Can you work these out from the model? Positions are in its coordinate system, mm. Round coordinates to 2 decimals unless told otherwise and drop trailing zeros. Order: outer loops, then holes, each group sorted by start corner. A loop starts at its lowest first (then second) coordinate and runs counter-clockwise, first axis right, second up.
Q1. If we section it at A-A (y = 68): Please give me the cut outline in (x, z), plus the area to 3 significant figures.
Q2. If we section it at D-D (x = 195): Please give me the cut outline in (y, z), plus the area to 3 significant figures.
Q3. If we section it at C-C (z = 4.5): Count the separate pieces of the cut face and the enclosed holes in it, plus the area to 3 significant figures.
Q4. If we section it at B-B (y = 10): Please give me the cut outline in (x, z).
Q5. If I drill on line 1 (Y direction, x = 30, z = 8.75); line 2 (X direction, y = 150, z = 2.5); line 3 (Y direction, x = 71.5, z = 11.5), over which ranges is the centre line in solid material (lowest first)?
Q6. Will this pin go through, and if not, where does the flat tip stop? P1, Ø3, axis at x = 30, y = 120, coming from the +Z side.
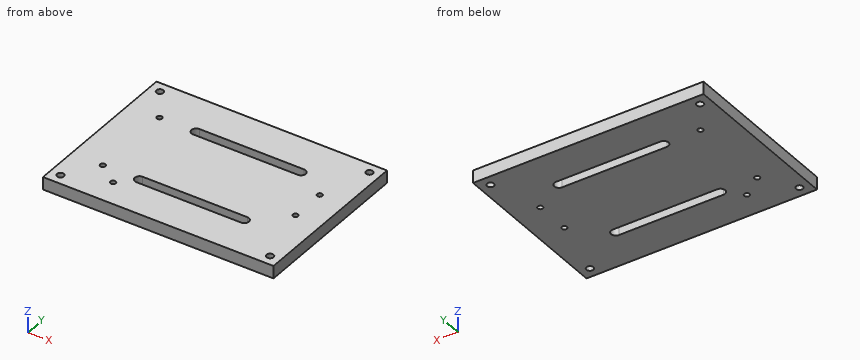
from build123d import *

# Parameters (mm, degrees)
SKETCH_1_W                  = 220
SKETCH_1_H                  = 160
SKETCH_1_R                  = 3.3
SKETCH_1_R_2                = 2.5
BASE_PLATE_220X160X12_DEPTH = 12


with BuildPart() as part:
    # 草图1 → Base_plate_220x160x12 (new body)
    with BuildSketch(Plane.XY):
        with Locations((110, 80)):
            Rectangle(SKETCH_1_W, SKETCH_1_H)
        with Locations((10, 10)):
            Circle(SKETCH_1_R, mode=Mode.SUBTRACT)
        with Locations((10, 150)):
            Circle(SKETCH_1_R, mode=Mode.SUBTRACT)
        with Locations((210, 10)):
            Circle(SKETCH_1_R, mode=Mode.SUBTRACT)
        with Locations((210, 150)):
            Circle(SKETCH_1_R, mode=Mode.SUBTRACT)
        with Locations((30, 40)):
            Circle(SKETCH_1_R_2, mode=Mode.SUBTRACT)
        with Locations((30, 120)):
            Circle(SKETCH_1_R_2, mode=Mode.SUBTRACT)
        with Locations((50, 25)):
            Circle(SKETCH_1_R_2, mode=Mode.SUBTRACT)
        with Locations((195, 68)):
            Circle(SKETCH_1_R_2, mode=Mode.SUBTRACT)
        with Locations((195, 102)):
            Circle(SKETCH_1_R_2, mode=Mode.SUBTRACT)
        with BuildLine():
            Line((65, 44.5), (165, 44.5))
            ThreePointArc((165, 44.5), (169.5, 40), (165, 35.5))
            Line((165, 35.5), (65, 35.5))
            ThreePointArc((65, 35.5), (60.5, 40), (65, 44.5))
        make_face(mode=Mode.SUBTRACT)
        with BuildLine():
            Line((65, 124.5), (165, 124.5))
            ThreePointArc((165, 124.5), (169.5, 120), (165, 115.5))
            Line((165, 115.5), (65, 115.5))
            ThreePointArc((65, 115.5), (60.5, 120), (65, 124.5))
        make_face(mode=Mode.SUBTRACT)
    extrude(amount=BASE_PLATE_220X160X12_DEPTH)


solid = part.part
Solution:
1. outline: (0, 0) - (192.5, 0) - (192.5, 12) - (0, 12) - close; (197.5, 0) - (220, 0) - (220, 12) - (197.5, 12) - close
1. area: 2,580 mm2
2. outline: (0, 0) - (65.5, 0) - (65.5, 12) - (0, 12) - close; (70.5, 0) - (99.5, 0) - (99.5, 12) - (70.5, 12) - close; (104.5, 0) - (160, 0) - (160, 12) - (104.5, 12) - close
2. area: 1,800 mm2
3. separate pieces: 1
3. enclosed holes: 11
3. area: 33,000 mm2
4. outline: (0, 0) - (6.7, 0) - (6.7, 12) - (0, 12) - close; (13.3, 0) - (206.7, 0) - (206.7, 12) - (13.3, 12) - close; (213.3, 0) - (220, 0) - (220, 12) - (213.3, 12) - close
5. line 1: y = 0 to 37.5, 42.5 to 117.5, 122.5 to 160
5. line 2: x = 0 to 6.7, 13.3 to 206.7, 213.3 to 220
5. line 3: y = 0 to 35.5, 44.5 to 115.5, 124.5 to 160
6. P1: passes through
